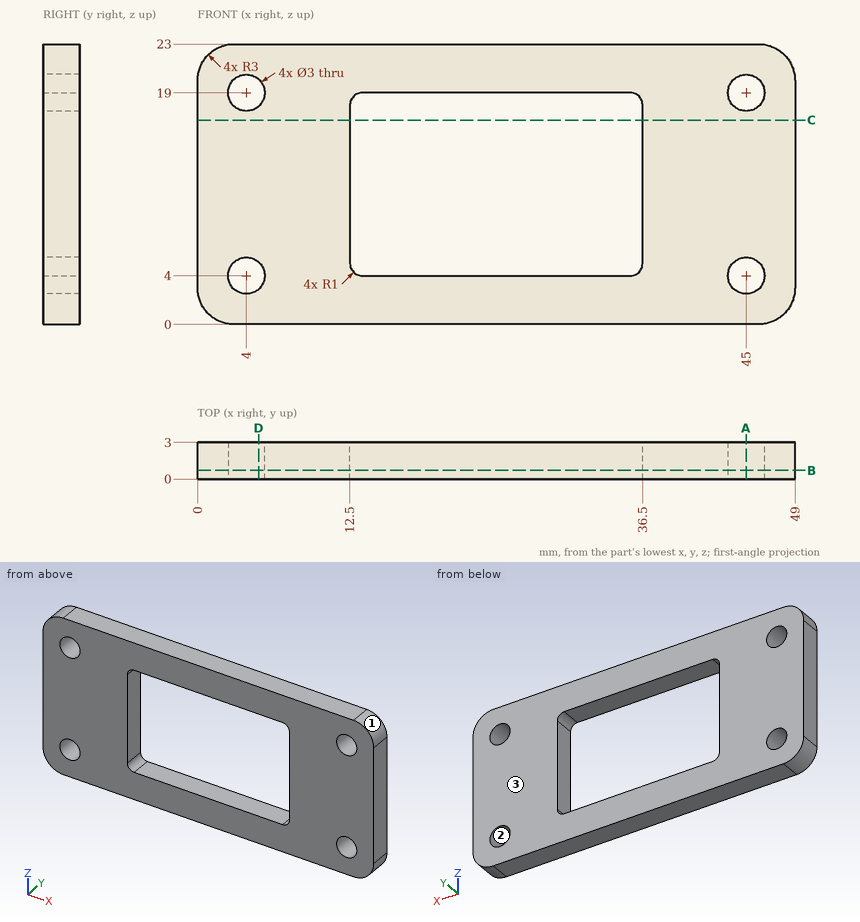
Geometry check sheet. Reference: drawing and pictorial views, mm from the part's lowest x, y, z. Coordinates: 2 decimals unless noted, no trailing zeros. Order: outer loops, then holes, each group sorted by start corner. A loop starts at its lowest first (then second) coordinate and runs counter-clockwise, first axis right, second up. Notation, with made-up numbers: (48.25, 87.25) - (101.25, 87.25) arc R31 ccw to (101.25, 115.25) - close; hole circle Ø10 at (-20.5, 69). An arc over 180 degrees is marked (long way). Answer in a Markdown table with one row per item. Add a question column.
1) Cross-section at C-C, the plane z = 16.75. Record the cut outline in (x, y).
2) Cross-section at D-D, the plane x = 5. Record the cut outline in (y, z).
3) Cross-section at A-A, the plane x = 45. Record the cut outline in (y, z).
4) Release check for a two-part mould opening along Z. For the marked faces 1, 2 and 3 record: +Z half, -Z half, draft (parallel to the pull), parting line (faces both ways), or undercut.
5) Cross-section at B-B, the plane y = 0.7. Record the cut outline in (x, z).
6) Material ranges on line 1 along Z through (x, y) = (45, 2.05); line 2 along X through (y, z) = (1.45, 11.75); line 3 along X through (y, z) = (1.2, 18), recorded low to high. Write a range as [from, to].
7) Gauge pin test, flat end, axial feed: P1, Ø2.5, axis at x = 4, z = 19, coming from the +Y side. Record the tip position at first contact, or that the pin passes through.
Check result:
| question | item | result |
|---|---|---|
| 1 | outline | (0, 0) - (12.5, 0) - (12.5, 3) - (0, 3) - close; (36.5, 0) - (49, 0) - (49, 3) - (36.5, 3) - close |
| 2 | outline | (0, 0) - (3, 0) - (3, 2.88) - (0, 2.88) - close; (0, 5.12) - (3, 5.12) - (3, 17.88) - (0, 17.88) - close; (0, 20.12) - (3, 20.12) - (3, 23) - (0, 23) - close |
| 3 | outline | (0, 0) - (3, 0) - (3, 2.5) - (0, 2.5) - close; (0, 5.5) - (3, 5.5) - (3, 17.5) - (0, 17.5) - close; (0, 20.5) - (3, 20.5) - (3, 23) - (0, 23) - close |
| 4 | face 1 | +Z half |
| 4 | face 2 | undercut |
| 4 | face 3 | draft |
| 5 | outline | (0, 3) arc R3 ccw to (3, 0) - (46, 0) arc R3 ccw to (49, 3) - (49, 20) arc R3 ccw to (46, 23) - (3, 23) arc R3 ccw to (0, 20) - close; hole circle Ø3 at (4, 4); hole circle Ø3 at (4, 19); hole (12.5, 5) arc R1 ccw to (13.5, 4) - (35.5, 4) arc R1 ccw to (36.5, 5) - (36.5, 18) arc R1 ccw to (35.5, 19) - (13.5, 19) arc R1 ccw to (12.5, 18) - close; hole circle Ø3 at (45, 4); hole circle Ø3 at (45, 19) |
| 6 | line 1 | z = [0, 2.5], [5.5, 17.5], [20.5, 23] |
| 6 | line 2 | x = [0, 12.5], [36.5, 49] |
| 6 | line 3 | x = [0, 2.88], [5.12, 12.5], [36.5, 43.88], [46.12, 49] |
| 7 | P1 | passes through |
